Autodesk Inventor part; units mm, degrees
ref_plane "YZ Plane" through (0, 0, 0) normal (1, 0, 0) x (0, 1, 0)
ref_plane "XZ Plane" through (0, 0, 0) normal (0, 1, 0) x (-1, 0, 0)
ref_plane "XY Plane" through (0, 0, 0) normal (0, 0, 1) x (1, 0, 0)
sketch "Stack Sketch" plane through (0, 0, 0) normal (0, 0, 1) x (1, 0, 0)
  line L0 (0, 0) -> (6.35, 0)
  line L1 (6.35, 0) -> (6.35, 6.35)
  line L2 (6.35, 6.35) -> (15.875, 38.1)
  line L3 (0, 44.45) -> (0, 0)
  line L4 (15.875, 38.1) -> (15.875, 46.0795) construction
  line L5 (15.875, 38.1) -> (14.1735, 44.45)
  line L6 (14.1735, 44.45) -> (0, 44.45)
  dimension "d0" = 6.35
  dimension "d1" = 38.1
  dimension "d5" = 6.35
  dimension "d6" = 44.45
  dimension "d7" = 15
  dimension "d17" = 15.875
revolve "Stack Revolve" add sketch "Stack Sketch" angle 360 about axis through (0, 44.45, 0) along (0, -1, 0)
sketch "Stack Hole Sketch" plane through (0, 44.45, 0) normal (0, 1, 0) x (1, 0, 0)
  point P0 (0, 0)
  point P1 (0, 0)
hole "Stack Hole" at (0, 44.45, 0) direction (0, -1, 0) diameter 9.525 depth 38.1 counterbore diameter 22.225 counterbore depth 9.525
chamfer "Bottom Chamfer" distance 0.254 angle 45 1 edges at (-6.35, 0, 0)
properties part number "Caufield_Stack"
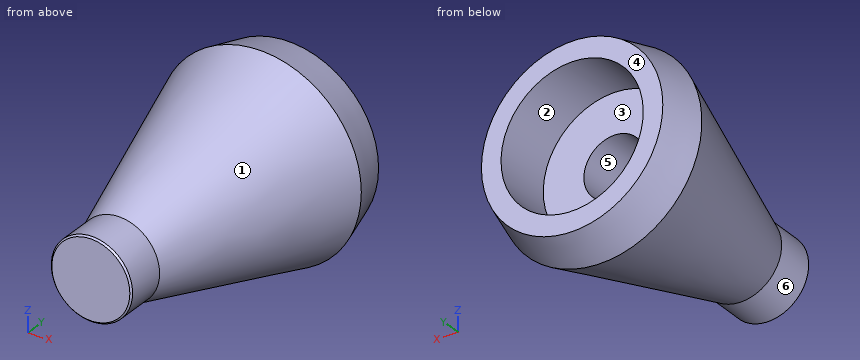
Design review of the part built by this model. Coordinates are the model's own, in mm. Face numbers are marked on the shaded views. A direction names the side the tool comes from. Coordinates: 2 decimals unless noted, no trailing zeros. Write each loop counter-clockwise with the first axis right and the second up, starting at its lowest first coordinate (ties: lowest second). Pieces come first, ordered by that corner, then holes. Notation, with made-up numbers: (23, 16) - (59, 16) arc R9 cw to (59, 27) - close; hole circle Ø1 at (-40, 34.5). An arc over 180 degrees is marked (long way). One line per item, written item: value.
1) Add section C-C (y = 36). State the section outline as (x, z) points (1 decimal).
Answer sheet:
outline: circle Ø30.5 at (0, 0); hole circle Ø22.2 at (0, 0)
2) For the marked faces 1 and 2, list the 3-axis set-ups (+Z, -Z, +X, -X, +Y, -Y) from which the entire face can be reached by the end or side of a thin tool; tool diameter is ignored.
Answer sheet:
face 1: -Y
face 2: +Y
3) Add section D-D (y = 17). State the section outline as (x, z) points (1 decimal), plus the area to 3 significant figures.
Answer sheet:
outline: circle Ø19.1 at (0, 0); hole circle Ø9.5 at (0, 0)
area: 215 mm2
4) Mouldability with a two-part tool opening along X and no side actions: class the marked faces 3, 4, 5 and 6 as +X half, -X half, draft (parallel to the pull), parting line (faces both ways), or undercut.
Answer sheet:
face 3: undercut
face 4: draft
face 5: undercut
face 6: parting line
5) Insertion check: pin 1 (8 mm diameter, centred on x = -4, y = 11.5, fed in from +Z); pin 2 (12.5 mm diameter, centred on x = 0, z = 0, fed in from +Y) (3 decimals); pin 3 (6 mm diameter, centred on y = 10.5, z = -2.5, fed in from +X). Each pin has a flat end and moves straight along its axis. Give the tip position at first contact, or say it passes through.
Answer sheet:
pin 1: stops at z = 8.71
pin 2: stops at y = 34.925
pin 3: stops at x = 8.32
6) To check wall thickness, follow probe 1 along X at (y, z) = (37.25, 0); probe 2 along X at (y, z) = (41.5, -3); probe 3 along Y at (x, z) = (2, 1). State the ranges of each line that lie inside material, in increasing order.
Answer sheet:
probe 1: x = -15.62 to -11.11, 11.11 to 15.62
probe 2: x = -14.66 to -10.7, 10.7 to 14.66
probe 3: y = 0 to 6.35
